from build123d import *

# Parameters (mm, degrees)
SKETCH2_R            = 11
BOSS_EXTRUDE2_DEPTH  = 1.5
BOSS_EXTRUDE3_START  = -15
SKETCH3_R            = 11
SKETCH3_R_2          = 9.652
BOSS_EXTRUDE3_DEPTH  = 15
SKETCH4_W            = 3
SKETCH4_H            = 21.794494718
BOSS_EXTRUDE4_DEPTH  = 58
SKETCH11_R           = 8.5
BOSS_EXTRUDE11_DEPTH = 1
SKETCH8_R            = 5
BOSS_EXTRUDE6_DEPTH  = 10
SKETCH15_R           = 3.175
ENCODER_BED_DEPTH    = 6
FILLET5_R            = 10
FILLET7_R            = 5
SKETCH21_R           = 4
CUT_EXTRUDE6_DEPTH   = 2
SKETCH22_R           = 22
BOSS_EXTRUDE13_DEPTH = 3
SKETCH23_R           = 2.6
CUT_EXTRUDE7_DEPTH   = 3
CIRPATTERN1_COUNT    = 8
SKETCH24_R           = 1.6
CUT_EXTRUDE8_DEPTH   = 3
CIRPATTERN2_COUNT    = 8
FILLET8_R            = 10


with BuildPart() as part:
    # Sketch2 → Boss-Extrude2 (new body)
    with BuildSketch(Plane(origin=(0, 0, 0), x_dir=(-1, 0, 0), z_dir=(0, 1, 0))):
        with Locations(Location((0, 0, 0), (0, 0, 90))):
            Circle(SKETCH2_R)
    extrude(amount=-BOSS_EXTRUDE2_DEPTH)

    # Sketch3 → Boss-Extrude3 (add)
    with BuildSketch(Plane(origin=(0, 0, 0), x_dir=(-1, 0, 0), z_dir=(0, -1, 0)).offset(BOSS_EXTRUDE3_START)):
        with Locations(Location((0, 0, 0), (0, 0, 270))):
            Circle(SKETCH3_R)
        with Locations(Location((0, 0, 0), (0, 0, 90))):
            Circle(SKETCH3_R_2, mode=Mode.SUBTRACT)
    extrude(amount=BOSS_EXTRUDE3_DEPTH)

    # Sketch4 → Boss-Extrude4 (add)
    with BuildSketch(Plane.XZ.offset(1.5)):
        Rectangle(SKETCH4_W, SKETCH4_H)
    extrude(amount=BOSS_EXTRUDE4_DEPTH)

    # Sketch11 → Boss-Extrude11 (add)
    with BuildSketch(Plane(origin=(1.5, 0, 0), x_dir=(0, 0, -1), z_dir=(1, 0, 0))):
        with Locations(Location((0, -49.5, 0), (0, 0, 180))):
            Circle(SKETCH11_R)
    extrude(amount=BOSS_EXTRUDE11_DEPTH)

    # Sketch8 → Boss-Extrude6 (add)
    with BuildSketch(Plane.ZY.offset(-2.5)):
        with Locations((0, -49.5)):
            Circle(SKETCH8_R)
    extrude(amount=-BOSS_EXTRUDE6_DEPTH)

    # Sketch15 → encoder_bed (cut)
    with BuildSketch(Plane(origin=(12.5, 0, 0), x_dir=(0, 0, -1), z_dir=(1, 0, 0))):
        with Locations((0, -49.5)):
            Circle(SKETCH15_R)
    extrude(amount=-ENCODER_BED_DEPTH, mode=Mode.SUBTRACT)

    # Fillet5
    fillet5_edges = [part.edges().sort_by_distance(p)[0] for p in [
        (0, -59.5, 10.897247359),
        (0, -59.5, -10.897247359),
    ]]
    fillet(fillet5_edges, radius=FILLET5_R)

    # Fillet7
    # the kernel refuses this fillet: 5 mm, written as the material it adds along each edge
    with BuildSketch(Plane(origin=(1.5, -1.5, 10.897247359), x_dir=(0, -1, 0), z_dir=(0, 0, -1))) as fillet7_piece_1_section:
        with BuildLine():
            CenterArc((FILLET7_R, -FILLET7_R), FILLET7_R, 90, 90)
            Line((0, -FILLET7_R), (0, 0))
            Line((0, 0), (FILLET7_R, 0))
        make_face()
    fillet7_piece_1 = extrude(amount=21.794494718, mode=Mode.PRIVATE)
    fillet7_piece_1 = fillet7_piece_1 & Plane(origin=(0, -2.650343277, 0), x_dir=(0, 0, 1), z_dir=(0, 1, 0)) * Cylinder(11, 64, mode=Mode.PRIVATE)
    add(fillet7_piece_1)
    with BuildSketch(Plane(origin=(-1.5, -1.5, -10.897247359), x_dir=(0, -1, 0), z_dir=(0, 0, 1))) as fillet7_piece_2_section:
        with BuildLine():
            CenterArc((FILLET7_R, -FILLET7_R), FILLET7_R, 90, 90)
            Line((0, -FILLET7_R), (0, 0))
            Line((0, 0), (FILLET7_R, 0))
        make_face()
    fillet7_piece_2 = extrude(amount=21.794494718, mode=Mode.PRIVATE)
    fillet7_piece_2 = fillet7_piece_2 & Plane(origin=(0, -2.650343277, 0), x_dir=(0, 0, 1), z_dir=(0, 1, 0)) * Cylinder(11, 64, mode=Mode.PRIVATE)
    add(fillet7_piece_2)

    # Sketch21 → Cut-Extrude6 (cut)
    with BuildSketch(Plane(origin=(12.5, 0, 0), x_dir=(0, 0, -1), z_dir=(1, 0, 0))):
        with Locations((0, -49.5)):
            Circle(SKETCH21_R)
    extrude(amount=-CUT_EXTRUDE6_DEPTH, mode=Mode.SUBTRACT)

    # Sketch22 → Boss-Extrude13 (add)
    with BuildSketch(Plane.ZY.offset(1.5)):
        with Locations((0, -49.5)):
            Circle(SKETCH22_R)
    extrude(amount=-BOSS_EXTRUDE13_DEPTH)

    # Sketch23 → Cut-Extrude7 (cut)
    with BuildSketch(Plane.ZY.offset(1.5)):
        with Locations((0, -32)):
            Circle(SKETCH23_R)
    cut_extrude7 = extrude(amount=-CUT_EXTRUDE7_DEPTH, mode=Mode.SUBTRACT)

    # CirPattern1: Cut-Extrude7 ×8 about axis
    cirpattern1_axis = Axis((0, -49.5, 0), (1, 0, 0))
    for i in range(1, CIRPATTERN1_COUNT):
        add(cut_extrude7.rotate(cirpattern1_axis, i * 360 / CIRPATTERN1_COUNT), mode=Mode.SUBTRACT)

    # Sketch24 → Cut-Extrude8 (cut)
    with BuildSketch(Plane.ZY.offset(1.5)):
        with Locations((6.696960066, -33.332108181)):
            Circle(SKETCH24_R)
    cut_extrude8 = extrude(amount=-CUT_EXTRUDE8_DEPTH, mode=Mode.SUBTRACT)

    # CirPattern2: Cut-Extrude8 ×8 about axis
    cirpattern2_axis = Axis((0, -49.5, 0), (1, 0, 0))
    for i in range(1, CIRPATTERN2_COUNT):
        add(cut_extrude8.rotate(cirpattern2_axis, i * 360 / CIRPATTERN2_COUNT), mode=Mode.SUBTRACT)

    # Fillet8
    fillet8_edges = [part.edges().sort_by_distance(p)[0] for p in [
        (0, -30.388485146, -10.897247359),
        (0, -30.388485146, 10.897247359),
    ]]
    fillet(fillet8_edges, radius=FILLET8_R)


solid = part.part
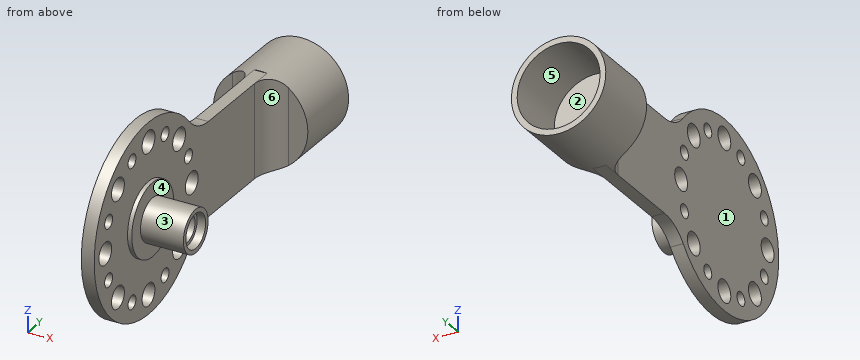
The model under review builds one solid part; all positions refer to its coordinate system, in mm. Face numbers are marked on the shaded views. A direction names the side the tool comes from. Coordinates: 2 decimals unless noted, no trailing zeros. Write each loop counter-clockwise with the first axis right and the second up, starting at its lowest first coordinate (ties: lowest second). Pieces come first, ordered by that corner, then holes. Notation, with made-up numbers: M 0,23.25 L 16,23.25 A16 cw 16,47.25 Z; hole C -20.75,77.25 d6. An arc over 180 degrees is marked long. Put each result on its own line as item: value.
1) Add section C-C on y = -8.5. Give the boundary of the cut face in (x, z), then the cut area to 3 significant figures.
Computed:
outline: M -1.5,-10.9 L 1.5,-10.9 L 1.5,10.9 L -1.5,10.9 Z
area: 65.4 mm2
2) Add section D-D on x = -4.25. Give the boundary of the cut face in (y, z).
Computed:
outline: M -2.03,-10.15 L 15,-10.15 L 15,-8.67 L 0,-8.67 L 0,8.67 L 15,8.67 L 15,10.15 L -2.03,10.15 Z
3) Wall thickness on probe 1 along Z at (x, y) = (-0.3, -49.5); probe 2 along X at (y, z) = (5.5, 0); probe 3 along Y at (x, z) = (10, -2.5): over which ranges is each line inside the solid? List them lowest first. Write a range as [from, to].
Computed:
probe 1: z = [-22, -20.1], [-14.9, 14.9], [20.1, 22]
probe 2: x = [-11, -9.65], [9.65, 11]
probe 3: y = [-53.83, -51.46], [-47.54, -45.17], [-1.5, 15]
4) Clearance check with flat-ended pins moving along their axes: pin 1 Ø8 at (y, z) = (-33.5, 16.5) entering from +X; pin 2 Ø3 at (y, z) = (-37.13, -12.37) entering from +X (3 decimals); pin 3 Ø22 at (y, z) = (-28, -10.5) entering from -X; pin 4 Ø1.3 at (x, z) = (-8.5, 0) entering from -Y. State where each tip first meets the part, or that it passes through.
Computed:
pin 1: stops at x = 1.5
pin 2: passes through
pin 3: stops at x = -1.5
pin 4: stops at y = -1.5
5) For the marked faces 4, 5 and 6, list the 3-axis set-ups (+Z, -Z, +X, -X, +Y, -Y) from which the entire face can be reached by the end or side of a thin tool; tool diameter is ignored.
Computed:
face 4: +X
face 5: +Y
face 6: +Z, -Z, +X
6) Add section A-A on x = 0. State how many separate pieces and enclosed holes the cut face has, then the cut area to 3 significant figures.
Computed:
separate pieces: 1
enclosed holes: 16
area: 1,950 mm2
7) Draft analysis for pull direction Y (two halves, no side actions). For the marked faces 1, 2 and 3, state which applies: released by +Y, released by -Y, zero draft, split by the parting line, or undercut.
Computed:
face 1: zero draft
face 2: released by +Y
face 3: undercut
